Source: CAD feature listing. Evaluate the final solid. Frame: model axes, mm. A direction names the side the tool comes from. Coordinates: 2 decimals unless noted, no trailing zeros. Loops run counter-clockwise (first coordinate to the right, second up) from the corner with the lowest first, then second, coordinate; pieces in that order, holes last.
Item 1: Pin query (flat end, axial travel): pin 1 Ø1.1 at (y, z) = (8.5, 11) entering from -X; pin 2 Ø1.5 at (y, z) = (5.78, -4.19) entering from -X; pin 3 Ø11.5 at (x, z) = (7.5, 2.5) entering from +Y. Return the tip coordinate at first contact, or that it passes through.
Item 2: Pull-direction query (Y, two-part tool) for faces 5 (the flat face through (18.6, 3.81, 6.1)), 6 (the flat face through (-1.095, 6.064, 4.54)), 7 (the cylindrical face through (3.054, 5.841, 12.603)); classes: +Y half, -Y half, draft (parallel to the pull), parting line (faces both ways), or undercut.
Item 3: Line query: probe 1 along X at (y, z) = (5.75, -1.75); probe 2 along Z at (x, y) = (17.5, 4); probe 3 along Y at (x, z) = (9.5, 13.5). Output: solid intervals per line, ascending.
Item 4: Reachability of faces 1 (the flat face through (12, 10.858, 14)), 2 (the flat face through (8, 11.557, 5)), 3 (the flat face through (2.159, 6, -3)), 4 (the flat face through (9.398, 6, -3)) from +Z, -Z, +X, -X, +Y, -Y: full face, straight path, thin tool, end or side. Return the list, or none.
Item 5: Section query A-A, the plane x = 16.5. Return the cut outline in (y, z).
Item 6: Section query B-B, the plane z = 8.75. Return the cut outline in (x, y) (3 decimals).
Item 7: Section query C-C, the plane y = -0.5. Return the cut outline in (x, z).
```python
from build123d import *

# Parameters (mm, degrees)
SKETCH1_W           = 17.145
SKETCH1_H           = 11.557
BOSS_EXTRUDE1_DEPTH = 10.541
SKETCH2_W           = 0.508
SKETCH2_H           = 4.699
BOSS_EXTRUDE2_DEPTH = 6.731
CUT_EXTRUDE1_REACH  = 24.017
SKETCH3_R           = 0.381
SKETCH4_W           = 20.828
SKETCH4_H           = 14.732
SKETCH4_W_2         = 14.364137932
SKETCH4_H_2         = 10.16
BOSS_EXTRUDE3_DEPTH = 2.032
CUT_EXTRUDE2_DEPTH  = 28.121934578
CUT_EXTRUDE3_DEPTH  = 28.652554914
BOSS_EXTRUDE4_DEPTH = 10.16
SKETCH8_W           = 3.055360255
SKETCH8_H           = 0.37050197
CUT_EXTRUDE4_DEPTH  = 0.4445
SKETCH9_R           = 1.410409678
SKETCH9_R_2         = 1.066337698
CUT_EXTRUDE5_DEPTH  = 0.4572
BOSS_EXTRUDE5_DEPTH = 4.445


with BuildPart() as part:
    # Sketch1 → Boss-Extrude1 (new body)
    with BuildSketch(Plane.XY):
        with Locations((8.5725, 5.7785)):
            Rectangle(SKETCH1_W, SKETCH1_H)
    extrude(amount=BOSS_EXTRUDE1_DEPTH)

    # Sketch2 → Boss-Extrude2 (add)
    with BuildSketch(Plane(origin=(0, 0, 0), x_dir=(-1, 0, 0), z_dir=(0, 0, -1))):
        with Locations((-1.905, 5.7785)):
            Rectangle(SKETCH2_W, SKETCH2_H)
        with Locations((-9.144, 5.7785)):
            Rectangle(SKETCH2_W, SKETCH2_H)
    extrude(amount=BOSS_EXTRUDE2_DEPTH)

    # Cut-Extrude1: up to this face of the body (flat: up to its plane)
    cut_extrude1_end = Plane(part.part.faces().sort_by_distance((9.398, 5.7785, -3.3655))[0])
    # Sketch3 → Cut-Extrude1 (cut, up to the picked face)
    with BuildSketch(Plane.ZY.offset(-1.651), mode=Mode.PRIVATE) as cut_extrude1_sk1:
        with Locations((-0.508, 5.7785)):
            Circle(SKETCH3_R)
    cut_extrude1_tool1 = split(extrude(cut_extrude1_sk1.sketch, amount=-CUT_EXTRUDE1_REACH, mode=Mode.PRIVATE), bisect_by=cut_extrude1_end, keep=Keep.BOTH, mode=Mode.PRIVATE)
    # Sketch3 → Cut-Extrude1 (cut, up to the picked face)
    with BuildSketch(Plane.ZY.offset(-1.651), mode=Mode.PRIVATE) as cut_extrude1_sk2:
        Polygon((-6.731, 6.604), (-5.207, 8.128), (-6.731, 8.128), align=None)
    cut_extrude1_tool2 = split(extrude(cut_extrude1_sk2.sketch, amount=-CUT_EXTRUDE1_REACH, mode=Mode.PRIVATE), bisect_by=cut_extrude1_end, keep=Keep.BOTH, mode=Mode.PRIVATE)
    # Sketch3 → Cut-Extrude1 (cut, up to the picked face)
    with BuildSketch(Plane.ZY.offset(-1.651), mode=Mode.PRIVATE) as cut_extrude1_sk3:
        Polygon((-6.731, 4.953), (-5.207, 3.429), (-6.731, 3.429), align=None)
    cut_extrude1_tool3 = split(extrude(cut_extrude1_sk3.sketch, amount=-CUT_EXTRUDE1_REACH, mode=Mode.PRIVATE), bisect_by=cut_extrude1_end, keep=Keep.BOTH, mode=Mode.PRIVATE)
    # Sketch3 → Cut-Extrude1 (cut, up to the picked face)
    with BuildSketch(Plane.ZY.offset(-1.651), mode=Mode.PRIVATE) as cut_extrude1_sk4:
        with BuildLine():
            ThreePointArc((-4.699, 5.3975), (-3.556, 5.7785), (-4.699, 6.1595))
            ThreePointArc((-4.699, 6.1595), (-5.08, 5.7785), (-4.699, 5.3975))
        make_face()
    cut_extrude1_tool4 = split(extrude(cut_extrude1_sk4.sketch, amount=-CUT_EXTRUDE1_REACH, mode=Mode.PRIVATE), bisect_by=cut_extrude1_end, keep=Keep.BOTH, mode=Mode.PRIVATE)
    add(cut_extrude1_tool1.solids().sort_by(Axis((1.651, 5.7785, -0.508), (1, 0, 0)))[0], mode=Mode.SUBTRACT)
    add(cut_extrude1_tool2.solids().sort_by(Axis((1.651, 7.62, -6.223), (1, 0, 0)))[0], mode=Mode.SUBTRACT)
    add(cut_extrude1_tool3.solids().sort_by(Axis((1.651, 3.937, -6.223), (1, 0, 0)))[0], mode=Mode.SUBTRACT)
    add(cut_extrude1_tool4.solids().sort_by(Axis((1.651, 5.7785, -4.272067), (1, 0, 0)))[0], mode=Mode.SUBTRACT)

    # Sketch4 → Boss-Extrude3 (add)
    with BuildSketch(Plane.XY.offset(10.541)):
        with Locations((8.5725, 5.7785)):
            Rectangle(SKETCH4_W, SKETCH4_H)
        with Locations((8.5725, 5.7785)):
            Rectangle(SKETCH4_W_2, SKETCH4_H_2, mode=Mode.SUBTRACT)
    extrude(amount=BOSS_EXTRUDE3_DEPTH)

    # Sketch5 → Cut-Extrude2 (cut, through all)
    with BuildSketch(Plane.XZ.offset(1.5875)):
        Polygon((-1.8415, 11.557), (0.1905, 12.573), (-1.8415, 12.573), align=None)
        Polygon((16.9545, 12.573), (18.9865, 11.557), (18.9865, 12.573), align=None)
    extrude(amount=-CUT_EXTRUDE2_DEPTH, mode=Mode.SUBTRACT)

    # Sketch6 → Cut-Extrude3 (cut, through all)
    with BuildSketch(Plane(origin=(18.9865, 0, 0), x_dir=(0, 0, -1), z_dir=(1, 0, 0))):
        Polygon((-11.557, 13.1445), (-12.573, 11.1125), (-12.573, 13.1445), align=None)
        Polygon((-11.557, -1.5875), (-12.573, -1.5875), (-12.573, 0.4445), align=None)
    extrude(amount=-CUT_EXTRUDE3_DEPTH, mode=Mode.SUBTRACT)

    # Sketch7 → Boss-Extrude4 (add)
    with BuildSketch(Plane.XZ.offset(-10.8585)):
        with BuildLine():
            Line((15.749219614, 10.541), (15.749219614, 12.573))
            add(Edge.make_bspline(
                [(15.749219614, 12.573), (14.476637744, 15.554000954), (11.939219614, 16.383)],
                knots=[0, 0, 0, 1, 1, 1], degree=2))
            add(Edge.make_bspline(
                [(11.939219614, 16.383), (9.824691935, 13.388087839), (1.390431034, 12.573)],
                knots=[0, 0, 0, 1, 1, 1], degree=2))
            Line((1.390431034, 12.573), (1.390431034, 10.541))
            Line((1.390431034, 10.541), (15.749219614, 10.541))
        make_face()
    extrude(amount=BOSS_EXTRUDE4_DEPTH)

    # Sketch8 → Cut-Extrude4 (cut)
    with BuildSketch(Plane(origin=(-4.022149692, 0, 6.488075329), x_dir=(-0.8499295023207375, 0, -0.5268964234883585), z_dir=(0.5268964234883585, 0, -0.8499295023207375))):
        with Locations((-16.095593607, 5.7785)):
            Rectangle(SKETCH8_W, SKETCH8_H)
    extrude(amount=CUT_EXTRUDE4_DEPTH, mode=Mode.SUBTRACT)

    # Sketch9 → Cut-Extrude5 (cut)
    with BuildSketch(Plane(origin=(-2.340608329, 0, 11.835119688), x_dir=(0.9809994846940211, 0, 0.1940103374309346), z_dir=(-0.1940103374309346, 0, 0.9809994846940211))):
        with Locations((6.849694399, 5.7785)):
            Circle(SKETCH9_R)
        with Locations((6.849694399, 5.7785)):
            Circle(SKETCH9_R_2, mode=Mode.SUBTRACT)
    extrude(amount=-CUT_EXTRUDE5_DEPTH, mode=Mode.SUBTRACT)

    # Sketch10 → Boss-Extrude5 (add)
    with BuildSketch(Plane(origin=(0, 8.255, 0), x_dir=(1, 0, 0), z_dir=(0, 1, 0))):
        Polygon((0, -10.541), (-2.159, -6.731), (0, -2.286), (0, -3.488132969), (-1.575106844, -6.731), (0, -9.510600313), align=None)
    boss_extrude5 = extrude(amount=-BOSS_EXTRUDE5_DEPTH)

    # Mirror1: Boss-Extrude5 across plane
    add(boss_extrude5.mirror(Plane(origin=(8.5725, 0, 0), x_dir=(0, 0, 1), z_dir=(1, 0, 0))))


solid = part.part
```
Verdict:
1. pin 1: stops at x = -1.84
1. pin 2: stops at x = 1.65
1. pin 3: stops at y = 11.56
2. face 5: -Y half
2. face 6: draft
2. face 7: undercut
3. probe 1: x = 1.65 to 2.16, 8.89 to 9.4
3. probe 2: z = 3.02 to 4.22, 8.88 to 9.91, 10.54 to 12.3
3. probe 3: y = 0.7 to 10.86
4. face 1: +Z, +X, -X, +Y
4. face 2: -Z, +X, -X, +Y
4. face 3: -Z, +Y, -Y
4. face 4: -Z, +X, +Y, -Y
5. outline: (-1.59, 10.54) - (0, 10.54) - (0, 0) - (11.56, 0) - (11.56, 10.54) - (13.14, 10.54) - (13.14, 11.56) - (11.11, 12.57) - (0.44, 12.57) - (-1.59, 11.56) - close
6. outline: (-1.015, 3.81) - (-0.431, 3.81) - (-0.431, 8.255) - (-1.015, 8.255) - close; (0, 0) - (17.145, 0) - (17.145, 11.557) - (0, 11.557) - close; (17.576, 3.81) - (18.16, 3.81) - (18.16, 8.255) - (17.576, 8.255) - close
7. outline: (-1.84, 10.54) - (18.99, 10.54) - (18.99, 11.56) - (17.9, 12.1) - (-0.75, 12.1) - (-1.84, 11.56) - close
